from build123d import *

# Parameters (mm, degrees)
BOSS_EXTRUDE1_DEPTH   = 11
M5_TAPPED_HOLE1_D     = 4.2
M5_TAPPED_HOLE1_DEPTH = 16.7381927
M5_TAPPED_HOLE1_TIP   = 1.2618073


with BuildPart() as part:
    # Sketch1 → Boss-Extrude1 (new body)
    with BuildSketch(Plane.XY):
        with BuildLine():
            Line((14, -15.93967455), (-14, -15.93967455))
            Line((-14, -15.93967455), (-14, -4.93967455))
            Line((-14, -4.93967455), (-10, -4.93967455))
            Line((-10, -4.93967455), (-9.5, -5.228349685))
            ThreePointArc((-9.5, -5.228349685), (-8.133974596, -4.862324281), (-8.5, -3.496298877))
            Line((-8.5, -3.496298877), (-9, -3.207623743))
            Line((-9, -3.207623743), (-9, 4.328274642))
            Line((-9, 4.328274642), (-8.5, 4.616949777))
            ThreePointArc((-8.5, 4.616949777), (-8.133974596, 5.982975181), (-9.5, 6.349000584))
            Line((-9.5, 6.349000584), (-10, 6.06032545))
            Line((-10, 6.06032545), (-14, 6.06032545))
            Line((-14, 6.06032545), (-14, 12.06032545))
            Line((-14, 12.06032545), (14, 12.06032545))
            Line((14, 12.06032545), (14, 6.06032545))
            Line((14, 6.06032545), (10, 6.06032545))
            Line((10, 6.06032545), (9.5, 6.349000584))
            ThreePointArc((9.5, 6.349000584), (8.133974596, 5.982975181), (8.5, 4.616949777))
            Line((8.5, 4.616949777), (9, 4.328274642))
            Line((9, 4.328274642), (9, -3.207623743))
            Line((9, -3.207623743), (8.5, -3.496298877))
            ThreePointArc((8.5, -3.496298877), (8.133974596, -4.862324281), (9.5, -5.228349685))
            Line((9.5, -5.228349685), (10, -4.93967455))
            Line((10, -4.93967455), (14, -4.93967455))
            Line((14, -4.93967455), (14, -15.93967455))
        make_face()
    extrude(amount=BOSS_EXTRUDE1_DEPTH)

    # M5 Tapped Hole1
    with Locations(Plane(origin=(0, -15.93967455, 0), x_dir=(-1, 0, 0), z_dir=(0, -1, 0))):
        with Locations((0, -5.5)):
            Hole(M5_TAPPED_HOLE1_D / 2, depth=M5_TAPPED_HOLE1_DEPTH)
            with Locations((0, 0, -(M5_TAPPED_HOLE1_DEPTH + M5_TAPPED_HOLE1_TIP / 2))):  # 118° drill point
                Cone(0, M5_TAPPED_HOLE1_D / 2, M5_TAPPED_HOLE1_TIP, mode=Mode.SUBTRACT)


solid = part.part
Design review of the part built by this model. Coordinates are the model's own, in mm. A direction names the side the tool comes from. Round coordinates to 2 decimals unless told otherwise and drop trailing zeros. Write each loop counter-clockwise with the first axis right and the second up, starting at its lowest first coordinate (ties: lowest second). Pieces come first, ordered by that corner, then holes. Notation, with made-up numbers: (-19, 13) - (17, 13) arc R26 cw to (17, 47) - close; hole circle Ø4 at (51, 88). An arc over 180 degrees is marked (long way). Return JSON: item names as keys, results as strings. Group by question number.
Item 1: The part is to be moulded in two halves that separate along X. For faces 6 (the face through (14, -10, 5)), 7 (the face through (8.1, -4.8, 5.4)), 8 (the face through (-9, 1, 5)), say which applies: pulls with the +X half, pulls with the -X half, needs draft (parallel to the pull), parting line crosses it, or undercut.
Item 2: Machinability: for faces 1 (the face through (0, -15.94, 3)), 2 (the face through (-12, -4.94, 5)), 3 (the face through (-14, -11, 5)), 4 (the face through (-0.46, -7.45, 7.55)), 5 (the face through (12, 6.06, 5)), which of the approach directions +Z, -Z, +X, -X, +Y, -Y give a long, thin tool a straight path to every point of the face, cutting with its end or side? Answer none if there is none.
Item 3: We need section C-C on z = 10. Write out the cut boundary in (x, y), and give its area (3 significant figures).
Item 4: We need section B-B on y = -1. Write out the cut boundary in (x, z), and give its area (3 significant figures).
Item 5: We need section A-A on x = -12. Write out the cut boundary in (y, z), and give its area (3 significant figures).
Item 6: We need section D-D on y = -8.5. Write out the cut boundary in (x, z).
Item 7: For probe 1 along Z at (x, y) = (0, -6); probe 2 along Y at (x, z) = (-12.25, 4); probe 3 along X at (y, z) = (-1.5, 10), list the stretches that pass through material, from the lowest coordinate up. Write a range as [from, to].
Item 8: Insertion check: P1, Ø1, axis at y = 0.5, z = 1.5, coming from the -X side; P2, Ø2.5, axis at y = -0.5, z = 6, coming from the +X side; P3, Ø2.5, axis at x = 0, z = 5.5, coming from the -Y side. Each pin has a flat end and moves straight along its axis. Give the tip position at first contact, or say it passes through.
Model answer:
{
 "1": {"face 6": "pulls with the +X half", "face 7": "undercut", "face 8": "pulls with the -X half"},
 "2": {"face 1": "+Z, -Z, +X, -X, -Y", "face 2": "+Z, -Z, -X", "face 3": "+Z, -Z, -X, +Y, -Y", "face 4": "-Y", "face 5": "+Z, -Z, +X"},
 "3": {"outline": "(-14, -15.94) - (14, -15.94) - (14, -4.94) - (10, -4.94) - (9.5, -5.23) arc R1 cw to (8.5, -3.5) - (9, -3.21) - (9, 4.33) - (8.5, 4.62) arc R1 cw to (9.5, 6.35) - (10, 6.06) - (14, 6.06) - (14, 12.06) - (-14, 12.06) - (-14, 6.06) - (-10, 6.06) - (-9.5, 6.35) arc R1 cw to (-8.5, 4.62) - (-9, 4.33) - (-9, -3.21) - (-8.5, -3.5) arc R1 cw to (-9.5, -5.23) - (-10, -4.94) - (-14, -4.94) - close", "area": "667 mm²"},
 "4": {"outline": "(-9, 0) - (9, 0) - (9, 11) - (-9, 11) - close; hole circle Ø4.2 at (0, 5.5)", "area": "184 mm²"},
 "5": {"outline": "(-15.94, 0) - (-4.94, 0) - (-4.94, 11) - (-15.94, 11) - close; (6.06, 0) - (12.06, 0) - (12.06, 11) - (6.06, 11) - close", "area": "187 mm²"},
 "6": {"outline": "(-14, 0) - (14, 0) - (14, 11) - (-14, 11) - close; hole circle Ø4.2 at (0, 5.5)"},
 "7": {"probe 1": "z = [0, 3.4], [7.6, 11]", "probe 2": "y = [-15.94, -4.94], [6.06, 12.06]", "probe 3": "x = [-9, 9]"},
 "8": {"P1": "stops at x = -9", "P2": "stops at x = 9", "P3": "stops at y = 1.31"}
}
